Geometry: final body of the model. Coordinates: model frame, mm. Face numbers are marked on the shaded views. A direction names the side the tool comes from. Give positions to 0.01 mm unless a question says otherwise; leave off trailing zeros. Order: outer loops, then holes, each group sorted by start corner. A loop starts at its lowest first (then second) coordinate and runs counter-clockwise, first axis right, second up. Notation, with made-up numbers: (84.25, -17) -> (142.25, -17) arc R38 ccw to (142.25, 21) -> close; hole circle Ø7 at (37.25, -31.75). An arc over 180 degrees is marked (long way). Answer in a Markdown table with one row per item. Add a question column.
Q1. Set-up query: the marked faces 1 and 2. Return all of +Z, -Z, +X, -X, +Y, -Y with unobstructed straight access to the full face (end or side cutting, diameter ignored); none if empty.
Q2. Contact query for flat-ended pins moving along their axis: P1, Ø7, axis at x = 104.5, y = 10.5, coming from the +Z side; P2, Ø4, axis at x = 7, z = 7, coming from the +Y side. Output: stop coordinate, or through.
Q3. Line query: line 1 along Z through (x, y) = (193, 0.4); line 2 along Z through (x, y) = (80, 0.6); line 3 along X through (y, z) = (0.65, 8). Output: solid intervals per line, ascending. Write a range as from..to.
Q4. Cut plane B-B on y = 7.5. Return the cut outline in (x, z), and give its area (3 significant figures).
Q5. Cut plane A-A on x = 187. Return the cut outline in (y, z), and give its area (3 significant figures).
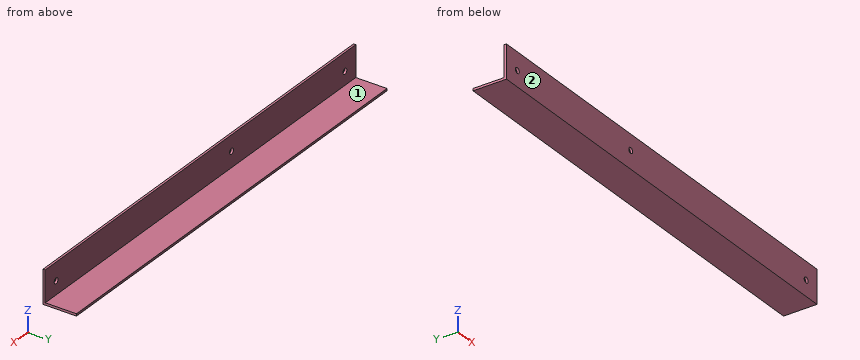
from build123d import *

# Parameters (mm, degrees)
SKETCH_1_W      = 200
SKETCH_1_H      = 15
EXTRUDE_1_DEPTH = 1
SKETCH_2_W      = 200
SKETCH_2_H      = 1
EXTRUDE_2_DEPTH = 14
M3X0_5_1_D      = 2.5
M3X0_5_2_D      = 2.5


with BuildPart() as part:
    # ｽｹｯﾁ1 → ﾎﾞｽ - 押し出し1 (new body)
    with BuildSketch(Plane.XY):
        with Locations((100, 7.5)):
            Rectangle(SKETCH_1_W, SKETCH_1_H)
    extrude(amount=EXTRUDE_1_DEPTH)

    # ｽｹｯﾁ2 → ﾎﾞｽ - 押し出し2 (add)
    with BuildSketch(Plane.XY.offset(1)):
        with Locations((100, 0.5)):
            Rectangle(SKETCH_2_W, SKETCH_2_H)
    extrude(amount=EXTRUDE_2_DEPTH)

    # M3x0.5 ねじ穴1 (through all)
    with Locations(Plane(origin=(0, 0, 0), x_dir=(-1, 0, 0), z_dir=(0, -1, 0))):
        with Locations((-193, -7)):
            m3x0_5_1 = Hole(M3X0_5_1_D / 2)

    # M3x0.5 ねじ穴2 (through all)
    with Locations(Plane(origin=(0, 1, 0), x_dir=(1, 0, 0), z_dir=(0, 1, 0))):
        with Locations((80, -8)):
            Hole(M3X0_5_2_D / 2)

    # ﾐﾗｰ1: M3x0.5 ねじ穴1 across plane
    add(m3x0_5_1.mirror(Plane(origin=(100, 0, 0), x_dir=(0, 0, 1), z_dir=(1, 0, 0))), mode=Mode.SUBTRACT)


solid = part.part
Completed:
| question | item | result |
|---|---|---|
| 1 | face 1 | +Z, +X, -X, +Y |
| 1 | face 2 | +Z, -Z, +X, -X, -Y |
| 2 | P1 | stops at z = 1 |
| 2 | P2 | stops at y = 1 |
| 3 | line 1 | z = 0..5.75, 8.25..15 |
| 3 | line 2 | z = 0..6.75, 9.25..15 |
| 3 | line 3 | x = 0..6.25, 7.75..78.75, 81.25..192.25, 193.75..200 |
| 4 | outline | (0, 0) -> (200, 0) -> (200, 1) -> (0, 1) -> close |
| 4 | area | 200 mm² |
| 5 | outline | (0, 0) -> (15, 0) -> (15, 1) -> (1, 1) -> (1, 15) -> (0, 15) -> close |
| 5 | area | 29.0 mm² |
